Verification items for the finished model (mm, model axes). A direction names the side the tool comes from. Round coordinates to 2 decimals unless told otherwise and drop trailing zeros. Loops run counter-clockwise (first coordinate to the right, second up) from the corner with the lowest first, then second, coordinate; pieces in that order, holes last. Notation, with made-up numbers: (78.25, 16.25) -> (94.25, 16.25) arc R14 cw to (94.25, 25.25) -> close; hole circle Ø1 at (42.5, 1). An arc over 180 degrees is marked (long way). Write item = value, one per line.
```python
from build123d import *

# Parameters (mm, degrees)
SKETCH1_W                      = 190
SKETCH1_H                      = 90
BOSS_EXTRUDE1_DEPTH            = 5
SKETCH2_W                      = 3.9
SKETCH2_H                      = 90
BOSS_EXTRUDE2_DEPTH            = 30
SKETCH3_W                      = 34
SKETCH3_H                      = 5
SKETCH3_W_2                    = 47
BOSS_EXTRUDE3_DEPTH            = 90
SKETCH4_W                      = 182.2
SKETCH4_H                      = 6
CUT_EXTRUDE1_DEPTH             = 5
CHAMFER6_SIZE                  = 20
BOSS_EXTRUDE4_DEPTH            = 78
FILLET5_R                      = 2
SKETCH9_R                      = 6.5
CUT_EXTRUDE4_DEPTH             = 10
SKETCH10_R                     = 7.55
CUT_EXTRUDE5_DEPTH             = 4
SKETCH15_R                     = 2.35
CUT_EXTRUDE7_DEPTH             = 8
CHAMFER7_SIZE                  = 1
SKETCH17_R                     = 6.1
CUT_EXTRUDE8_DEPTH             = 3.2
FILLET7_R                      = 0.2
CHAMFER8_SIZE                  = 9.9
CUT_EXTRUDE9_REACH             = 164.433
SKETCH18_W                     = 5
SKETCH18_H                     = 78
CUT_EXTRUDE9_DIRECTION_2_REACH = 164.433
BOSS_EXTRUDE5_DEPTH            = 78
FILLET8_R                      = 5
SKETCH21_W                     = 114.2
SKETCH21_H                     = 78
CUT_EXTRUDE10_DEPTH            = 3


with BuildPart() as part:
    # Sketch1 → Boss-Extrude1 (new body)
    with BuildSketch(Plane.XY):
        Rectangle(SKETCH1_W, SKETCH1_H)
    extrude(amount=BOSS_EXTRUDE1_DEPTH)

    # Sketch2 → Boss-Extrude2 (add)
    with BuildSketch(Plane.XY.offset(5)):
        with Locations((-93.05, 0)):
            Rectangle(SKETCH2_W, SKETCH2_H)
        with Locations((93.05, 0)):
            Rectangle(SKETCH2_W, SKETCH2_H)
    extrude(amount=BOSS_EXTRUDE2_DEPTH)

    # Sketch3 → Boss-Extrude3 (add)
    with BuildSketch(Plane(origin=(0, 45, 0), x_dir=(1, 0, 0), z_dir=(0, 1, 0))):
        with Locations((-74.1, -16.5)):
            Rectangle(SKETCH3_W, SKETCH3_H)
        with Locations((67.6, -16.5)):
            Rectangle(SKETCH3_W_2, SKETCH3_H)
    extrude(amount=-BOSS_EXTRUDE3_DEPTH)

    # Sketch4 → Cut-Extrude1 (cut)
    with BuildSketch(Plane.XY.offset(19)):
        with Locations((0, 42)):
            Rectangle(SKETCH4_W, SKETCH4_H)
        with Locations((0, -42)):
            Rectangle(SKETCH4_W, SKETCH4_H)
    extrude(amount=-CUT_EXTRUDE1_DEPTH, mode=Mode.SUBTRACT)

    # Chamfer6
    # the kernel refuses this chamfer: 20 mm, written as the material it adds along each edge
    with BuildSketch(Plane(origin=(-91.1, 45, 5), x_dir=(0.9996219169112968, 0, -0.02749587661058636), z_dir=(0, -1, 0))) as chamfer6_piece_1:
        Polygon((CHAMFER6_SIZE * 0.999621916911, CHAMFER6_SIZE * 0.0274958766106), (-CHAMFER6_SIZE * 0.0274958766106, CHAMFER6_SIZE * 0.999621916911), (0, 0), align=None)
    extrude(amount=90)
    with BuildSketch(Plane(origin=(91.1, -45, 5), x_dir=(0.027495876610586317, 0, 0.9996219169112968), z_dir=(0, 1, 0))) as chamfer6_piece_2:
        Polygon((CHAMFER6_SIZE * 0.999621916911, -CHAMFER6_SIZE * 0.0274958766106), (-CHAMFER6_SIZE * 0.0274958766106, -CHAMFER6_SIZE * 0.999621916911), (0, 0), align=None)
    extrude(amount=90)
    # the kernel refuses this chamfer: 20 mm, written as the material it takes off along each edge
    with BuildSketch(Plane(origin=(-95, -96.433659759, 0), x_dir=(0.9996219169112968, 0, -0.027495876610586372), z_dir=(0, 1, 0)), Plane(origin=(95, 96.433659759, 0), x_dir=(-0.9996219169112968, 0, -0.027495876610586372), z_dir=(0, -1, 0))) as chamfer6_2_piece_1:
        Polygon((CHAMFER6_SIZE * 0.999621916911, -CHAMFER6_SIZE * 0.0274958766106), (-CHAMFER6_SIZE * 0.0274958766106, -CHAMFER6_SIZE * 0.999621916911), (0, 0), align=None)
    extrude(amount=192.867319519, mode=Mode.SUBTRACT)

    # Sketch7 → Boss-Extrude4 (add)
    with BuildSketch(Plane(origin=(0, 39, 0), x_dir=(1, 0, 0), z_dir=(0, 1, 0))):
        Polygon((-85.1, -19), (-91.1, -25), (-91.1, -35), (-68.1, -35), (-68.1, -19), align=None)
        Polygon((68.1, -35), (68.1, -19), (85.1, -19), (91.1, -25), (91.1, -35), align=None)
    extrude(amount=-BOSS_EXTRUDE4_DEPTH)

    # Fillet5
    fillet5_edges = [part.edges().sort_by_distance(p)[0] for p in [
        (-68.1, 0, 35),
        (68.1, 0, 35),
    ]]
    fillet(fillet5_edges, radius=FILLET5_R)

    # Sketch9 → Cut-Extrude4 (cut)
    with BuildSketch(Plane.XY.offset(35)):
        with Locations((-82.45, -0.90743758)):
            Circle(SKETCH9_R)
        with Locations(Location((82.45, -0.90743758, 0), (0, 0, 180))):
            Circle(SKETCH9_R)
    extrude(amount=-CUT_EXTRUDE4_DEPTH, mode=Mode.SUBTRACT)

    # Sketch10 → Cut-Extrude5 (cut)
    with BuildSketch(Plane.XY.offset(35)):
        with Locations((-82.45, -0.90743758)):
            Circle(SKETCH10_R)
        with Locations((82.45, -0.90743758)):
            Circle(SKETCH10_R)
    extrude(amount=-CUT_EXTRUDE5_DEPTH, mode=Mode.SUBTRACT)

    # Sketch15 → Cut-Extrude7 (cut)
    with BuildSketch(Plane(origin=(0, 39, 0), x_dir=(1, 0, 0), z_dir=(0, 1, 0))):
        with Locations(Location((75.766666667, -21, 0), (0, 0, 270))):
            Circle(SKETCH15_R)
        with Locations(Location((-75.766666667, -21, 0), (0, 0, 90))):
            Circle(SKETCH15_R)
        with Locations(Location((78.766666667, -29, 0), (0, 0, 270))):
            Circle(SKETCH15_R)
        with Locations(Location((-78.766666667, -29, 0), (0, 0, 90))):
            Circle(SKETCH15_R)
    extrude(amount=-CUT_EXTRUDE7_DEPTH, mode=Mode.SUBTRACT)

    # Chamfer7
    chamfer7_edges = [part.edges().sort_by_distance(p)[0] for p in [
        (-75.766666667, 39, 23.35),
        (78.766666667, 39, 26.65),
        (-78.766666667, 39, 31.35),
        (75.766666667, 39, 18.65),
    ]]
    chamfer(chamfer7_edges, length=CHAMFER7_SIZE)

    # Sketch17 → Cut-Extrude8 (cut)
    with BuildSketch(Plane.XZ.offset(39)):
        with Locations((79.6, 27)):
            Circle(SKETCH17_R)
        with Locations(Location((-79.6, 27, 0), (0, 0, 180))):
            Circle(SKETCH17_R)
    extrude(amount=-CUT_EXTRUDE8_DEPTH, mode=Mode.SUBTRACT)

    # Fillet7
    fillet7_edges = [part.edges().sort_by_distance(p)[0] for p in [
        (73.5, -39, 27),
        (-73.5, -39, 27),
    ]]
    fillet(fillet7_edges, radius=FILLET7_R)

    # Chamfer8
    # the kernel refuses this chamfer: 9.9 mm, written as the material it takes off along each edge
    with BuildSketch(Plane(origin=(-95, 45, -5.459661581), x_dir=(0.9996219169112968, 0.027495876610586265, 0), z_dir=(0, 0, 1)), Plane(origin=(95, 45, 60.459661581), x_dir=(-0.9996219169112968, 0.02749587661058615, 0), z_dir=(0, 0, -1))) as chamfer8_piece_1:
        Polygon((CHAMFER8_SIZE * 0.999621916911, -CHAMFER8_SIZE * 0.0274958766106), (-CHAMFER8_SIZE * 0.0274958766106, -CHAMFER8_SIZE * 0.999621916911), (0, 0), align=None)
    extrude(amount=65.919323162, mode=Mode.SUBTRACT)

    # Cut-Extrude9: up to this face of the body (flat: up to its plane)
    cut_extrude9_end = Plane(part.part.faces().sort_by_distance((-68.1, 0, 26))[0])
    # Sketch18 → Cut-Extrude9 (cut, up to the picked face)
    with BuildSketch(Plane(origin=(-57.1, 0, 0), x_dir=(0, 0, -1), z_dir=(1, 0, 0)), mode=Mode.PRIVATE) as cut_extrude9_sk1:
        with Locations((-16.5, 0)):
            Rectangle(SKETCH18_W, SKETCH18_H)
    cut_extrude9_tool1 = split(extrude(cut_extrude9_sk1.sketch, amount=-CUT_EXTRUDE9_REACH, mode=Mode.PRIVATE), bisect_by=cut_extrude9_end, keep=Keep.BOTH, mode=Mode.PRIVATE)
    add(cut_extrude9_tool1.solids().sort_by(Axis((-57.1, 0, 16.5), (-1, 0, 0)))[0], mode=Mode.SUBTRACT)

    # Cut-Extrude9 direction 2: up to this face of the body (flat: up to its plane)
    cut_extrude9_direction_2_end = Plane(part.part.faces().sort_by_distance((68.1, 0, 26))[0])
    # Sketch18 → Cut-Extrude9 direction 2 (cut, up to the picked face)
    with BuildSketch(Plane(origin=(-57.1, 0, 0), x_dir=(0, 0, -1), z_dir=(1, 0, 0)), mode=Mode.PRIVATE) as cut_extrude9_direction_2_sk1:
        with Locations((-16.5, 0)):
            Rectangle(SKETCH18_W, SKETCH18_H)
    cut_extrude9_direction_2_tool1 = split(extrude(cut_extrude9_direction_2_sk1.sketch, amount=CUT_EXTRUDE9_DIRECTION_2_REACH, mode=Mode.PRIVATE), bisect_by=cut_extrude9_direction_2_end, keep=Keep.BOTH, mode=Mode.PRIVATE)
    add(cut_extrude9_direction_2_tool1.solids().sort_by(Axis((-57.1, 0, 16.5), (1, 0, 0)))[0], mode=Mode.SUBTRACT)

    # Sketch20 → Boss-Extrude5 (add)
    with BuildSketch(Plane(origin=(0, 39, 0), x_dir=(1, 0, 0), z_dir=(0, 1, 0))):
        Polygon((-68.1, -14), (-68.1, -5), (-71.1, -5), (-80.1, -14), align=None)
        Polygon((71.1, -5), (80.1, -14), (68.1, -14), (68.1, -5), align=None)
    extrude(amount=-BOSS_EXTRUDE5_DEPTH)

    # Fillet8
    fillet8_edges = [part.edges().sort_by_distance(p)[0] for p in [
        (-68.1, 0, 5),
        (68.1, 0, 5),
    ]]
    fillet(fillet8_edges, radius=FILLET8_R)

    # Sketch21 → Cut-Extrude10 (cut)
    with BuildSketch(Plane.XY.offset(5)):
        Rectangle(SKETCH21_W, SKETCH21_H)
    extrude(amount=-CUT_EXTRUDE10_DEPTH, mode=Mode.SUBTRACT)


solid = part.part
```
(1) Sectioned sample at A-A, the plane z = 15. Record the cut outline in (x, y).
Filled sheet:
outline = (-90, -45) -> (-81.1, -45) -> (-81.1, -39) -> (-68.1, -39) -> (-68.1, 39) -> (-81.1, 39) -> (-81.1, 45) -> (-85.1, 45) -> (-90, 40.1) -> close; (68.1, -39) -> (81.1, -39) -> (81.1, -45) -> (90, -45) -> (90, 40.1) -> (85.1, 45) -> (81.1, 45) -> (81.1, 39) -> (68.1, 39) -> close
(2) Material ranges on probe 1 along X at (y, z) = (33.25, 29); probe 2 along X at (y, z) = (-21, 24.5); probe 3 along X at (y, z) = (35.25, 29), recorded low to high. Write a range as from..to.
Filled sheet:
probe_1 = -95..-81.12, -76.42..-68.1, 68.1..76.42, 81.12..95
probe_2 = -95..-68.1, 68.1..95
probe_3 = -94.85..-81.12, -76.42..-68.1, 68.1..76.42, 81.12..94.85
(3) Sectioned sample at D-D, the plane z = 29. Count the separate pieces of the cut face and the enclosed holes in it, and give its area (3 significant figures).
Filled sheet:
separate_pieces = 2
enclosed_holes = 2
area = 3,810 mm2
(4) Draft check along Z on faces 1 (the face through (-90, -1, 33)), 2 (the face through (-66.67, -0.55, 6.5)), 3 (the face through (77.867, 34.549, 31.171)), 4 (the face through (-80, -35.8, 27)). Enter one of: released by +Z, released by -Z, zero draft, split by the parting line, or undercut.
Filled sheet:
face_1 = zero draft
face_2 = released by +Z
face_3 = undercut
face_4 = undercut
(5) Go/stop test with flat-tipped pins: pin 1 Ø10 at (x, z) = (77, 28.5) entering from -Y; pin 2 Ø10 at (x, y) = (-10, 6) entering from +Z; pin 3 Ø5 at (x, z) = (77.5, 28.5) entering from +Y. Record where each tip stops, or that it passes through.
Filled sheet:
pin_1 = -39
pin_2 = 2
pin_3 = 39
(6) Sectioned sample at C-C, the plane x = 50. Record the cut outline in (y, z), and give its area (3 significant figures).
Filled sheet:
outline = (-45, 0) -> (45, 0) -> (45, 5) -> (39, 5) -> (39, 2) -> (-39, 2) -> (-39, 5) -> (-45, 5) -> close
area = 216 mm2
(7) Set-up check for faces 5 (the face through (-68.1, 1, 22)), 6 (the face through (-77, -39, 20)), 7 (the face through (83, -1, 25)), 8 (the face through (-79, 31, 29)): record each of +Z, -Z, +X, -X, +Y, -Y from which the full face is reachable in a straight line by a thin tool's end or side.
Filled sheet:
face_5 = +Z, +Y, -Y
face_6 = +Z, -Y
face_7 = +Z
face_8 = +Y
(8) Sectioned sample at B-B, the plane y = -33. Record the cut outline in (x, z), and give its area (3 significant figures).
Filled sheet:
outline = (-95, 20) -> (-75, 0) -> (75, 0) -> (95, 20) -> (95, 35) -> (70.1, 35) arc R2 ccw to (68.1, 33) -> (68.1, 10) arc R5 cw to (63.1, 5) -> (57.1, 5) -> (57.1, 2) -> (-57.1, 2) -> (-57.1, 5) -> (-63.1, 5) arc R5 cw to (-68.1, 10) -> (-68.1, 33) arc R2 ccw to (-70.1, 35) -> (-95, 35) -> close
area = 1,830 mm2
